Read the model definition and answer for the solid it produces. Units are mm, in the model's axes. Round coordinates to 2 decimals unless told otherwise and drop trailing zeros. Write each loop counter-clockwise with the first axis right and the second up, starting at its lowest first coordinate (ties: lowest second). Pieces come first, ordered by that corner, then holes. Notation, with made-up numbers: (26, 63) - (80, 63) arc R20 cw to (80, 92) - close; hole circle Ø5 at (58.25, -39). An arc over 180 degrees is marked (long way). One line per item, written item: value. Start each with the question number.
(1) A cutting plane is placed at A-A, the plane x = 3.5. Determine the outline of the cut face in (y, z), plus the area to 3 significant figures.
(2) A flat-ended cylindrical pin translates along its axis: pin 1 Ø2.5 at (x, z) = (-3.5, 0) entering from -Y. Find the tip coordinate at first contact, or state that the pin passes through.
(3) A cutting plane is placed at C-C, the plane y = -0.2. Determine the outline of the cut face in (x, z), plus the area to 3 significant figures.
(4) Find the intervals of material crossed by L1, parallel to X at y = -2.4, z = -0.05; L2, parallel to Z at x = 3.5, y = -1.9; L3, parallel to X at y = -2.25, z = -0.65, in increasing order.
(5) A cutting plane is placed at B-B, the plane z = 0. Determine the outline of the cut face in (x, y).
(6) A cutting plane is placed at D-D, the plane z = -1.2. Determine the outline of the cut face in (x, y), plus the area to 3 significant figures.
(7) The mould has two halves that part along Z. Classify faces 1 (the face through (-2.114, -1.369, -0.575)), 2 (the face through (0, 0, 0)), 3 (the face through (0, -1, -2.25)): +Z half, -Z half, draft (parallel to the pull), parting line (faces both ways), or undercut.
from build123d import *

# Parameters (mm, degrees)
F0_W     = 12
F0_H     = 4.5
F1_DEPTH = 2.7
F2_R     = 1.5
F3_DEPTH = 25


with BuildPart() as f1:
    # F0 (on Front) → F1 (new body)
    with BuildSketch(Plane.XZ):
        Rectangle(F0_W, F0_H)
    extrude(amount=F1_DEPTH)

    # F2 (on face) → F3 (cut)
    with BuildSketch(Plane.XZ.offset(2.7)):
        with Locations((-3.5, 0)):
            Circle(F2_R)
        with BuildLine():
            ThreePointArc((5, 0), (3.5, 1.5), (2, 0))
            ThreePointArc((2, 0), (3.5, -1.5), (5, 0))
        make_face()
    extrude(amount=-F3_DEPTH, mode=Mode.SUBTRACT)


solid = f1.part
Here are the results:
1. outline: (-2.7, -2.25) - (0, -2.25) - (0, -1.5) - (-2.7, -1.5) - close; (-2.7, 1.5) - (0, 1.5) - (0, 2.25) - (-2.7, 2.25) - close
1. area: 4.05 mm²
2. pin 1: through
3. outline: (-6, -2.25) - (6, -2.25) - (6, 2.25) - (-6, 2.25) - close; hole circle Ø3 at (-3.5, 0); hole circle Ø3 at (3.5, 0)
3. area: 39.9 mm²
4. L1: -6 to -5, -2 to 2, 5 to 6
4. L2: -2.25 to -1.5, 1.5 to 2.25
4. L3: -6 to -4.85, -2.15 to 2.15, 4.85 to 6
5. outline: (-6, -2.7) - (-5, -2.7) - (-5, 0) - (-6, 0) - close; (-2, -2.7) - (2, -2.7) - (2, 0) - (-2, 0) - close; (5, -2.7) - (6, -2.7) - (6, 0) - (5, 0) - close
6. outline: (-6, -2.7) - (-4.4, -2.7) - (-4.4, 0) - (-6, 0) - close; (-2.6, -2.7) - (2.6, -2.7) - (2.6, 0) - (-2.6, 0) - close; (4.4, -2.7) - (6, -2.7) - (6, 0) - (4.4, 0) - close
6. area: 22.7 mm²
7. face 1: undercut
7. face 2: draft
7. face 3: -Z half
